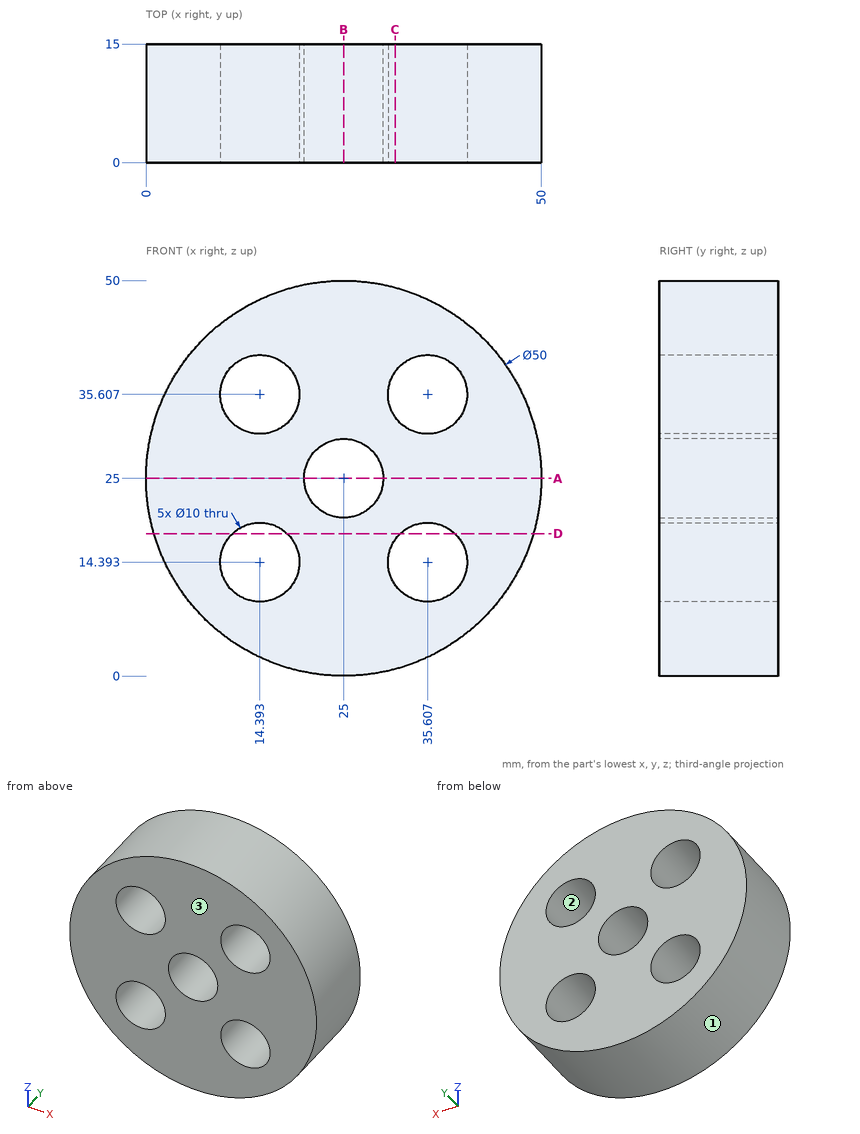
Answer from the drawing. Dimensions are ordinates in mm from the lowest x, y and z of the part. Give positions to 0.01 mm unless a question says otherwise; leave off trailing zeros. Order: outer loops, then holes, each group sorted by start corner. A loop starts at its lowest first (then second) coordinate and runs counter-clockwise, first axis right, second up. Notation, with made-up numbers: (54, 72.5) -> (102, 72.5) arc R29 ccw to (102, 92.5) -> close; hole circle Ø9 at (61, -23.5). An arc over 180 degrees is marked (long way). Answer as a JSON object with one key per item and string values. Group by question number.
1. Consider line 1 along X through (y, z) = (5, 33) (1 decimal); line 2 along X through (y, z) = (12.5, 39) (1 decimal); line 3 along Z through (x, y) = (16, 14.25) (1 decimal). Determine where each line is inside the solid, lowest interval first. Write a range as [from, to].
2. Flat-ended cylindrical pins translate along their axes: pin 1 Ø4 at (x, y) = (28.5, 11) entering from -Z (1 decimal); pin 2 Ø4 at (x, y) = (14.5, 12) entering from +Z; pin 3 Ø4 at (x, y) = (34.5, 11.5) entering from +Z. Find the tip coordinate at first contact, or state that the pin passes through.
3. The mould has two halves that part along Z. Classify the marked faces 1, 2 and 3: released by +Z, released by -Z, zero draft, split by the parting line, or undercut.
4. Section C-C on x = 31.5 is taken. Determine the outline of the cut face in (y, z) (1 decimal), plus the area to 3 significant figures.
5. Section A-A on z = 25 is taken. Determine the outline of the cut face in (x, y).
6. Section B-B on x = 25 is taken. Determine the outline of the cut face in (y, z).
7. Section D-D on z = 18 is taken. Determine the outline of the cut face in (x, y).
Result sheet:
{
 "1": {"line 1": "x = [1.3, 10.1], [18.7, 31.3], [39.9, 48.7]", "line 2": "x = [4.3, 10.7], [18.1, 31.9], [39.3, 45.7]", "line 3": "z = [1.7, 9.7], [19.1, 30.9], [40.3, 48.3]"},
 "2": {"pin 1": "stops at z = 0", "pin 2": "stops at z = 48.51", "pin 3": "stops at z = 48.85"},
 "3": {"face 1": "split by the parting line", "face 2": "undercut", "face 3": "zero draft"},
 "4": {"outline": "(0, 0.9) -> (15, 0.9) -> (15, 11.5) -> (0, 11.5) -> close; (0, 17.2) -> (15, 17.2) -> (15, 32.8) -> (0, 32.8) -> close; (0, 38.5) -> (15, 38.5) -> (15, 49.1) -> (0, 49.1) -> close", "area": "553 mm^2"},
 "5": {"outline": "(0, 0) -> (20, 0) -> (20, 15) -> (0, 15) -> close; (30, 0) -> (50, 0) -> (50, 15) -> (30, 15) -> close"},
 "6": {"outline": "(0, 0) -> (15, 0) -> (15, 20) -> (0, 20) -> close; (0, 30) -> (15, 30) -> (15, 50) -> (0, 50) -> close"},
 "7": {"outline": "(1, 0) -> (10.93, 0) -> (10.93, 15) -> (1, 15) -> close; (17.86, 0) -> (32.14, 0) -> (32.14, 15) -> (17.86, 15) -> close; (39.07, 0) -> (49, 0) -> (49, 15) -> (39.07, 15) -> close"}
}
